Here's how the part is built. I have some questions about the finished solid (model axes, mm). Face numbers are marked on the shaded views. A direction names the side the tool comes from. Coordinates: 2 decimals unless noted, no trailing zeros. Write each loop counter-clockwise with the first axis right and the second up, starting at its lowest first coordinate (ties: lowest second). Pieces come first, ordered by that corner, then holes. Notation, with made-up numbers: M 35.25,24.25 L 58.25,24.25 A17 cw 58.25,42.25 Z; hole C 68,65 d2. An arc over 180 degrees is marked long. Use one line per item in the form item = value. Start each with the question number.
1. I'm going to push flat-ended pins straight in: pin 1 Ø5 at (x, y) = (365, -1) entering from +Z; pin 2 Ø3 at (x, z) = (369.5, 5.5) entering from -Y; pin 3 Ø3 at (x, z) = (371.5, 0.5) entering from -Y; pin 4 Ø3 at (x, y) = (354, -3.5) entering from +Z. Where does each tip first touch, or does it pass through?
2. On a 3-axis mill with a long thin cutter (end or side, diameter ignored), from which of +Z, -Z, +X, -X, +Y, -Y can I reach the whole of each face in a straight line? I mean the marked faces 5, 6 and 7. Say none if no direction works.
3. I want a section at B-B, the plane x = 351.5. List the corners of the cut face in (y, z) for me, plus the area to 3 significant figures.
4. I want a section at C-C, the plane x = 344. List the corners of the cut face in (y, z) for me, plus the area to 3 significant figures.
5. Thinking about a two-plate mould opening in Z: for the marked faces 1, 2, 3 and 4, which applies, released by +Z, released by -Z, zero draft, split by the parting line, or undercut?
6. Please list where these lines run through material, in increasing order: line 1 along X through (y, z) = (0, 0); line 2 along Y through (x, z) = (339.25, 0); line 3 along X through (y, z) = (1.75, -4.5). Write a range as [from, to].
7. I want a section at A-A, the plane z = 0. Count the separate pieces of the cut face and the enclosed holes in it, plus the area to 3 significant figures.
from build123d import *

# Parameters (mm, degrees)
SKETCH1_R               = 143.51
BOSS_EXTRUDE1_DEPTH     = 50.8
SKETCH2_R               = 68.58
BOSS_EXTRUDE2_DEPTH     = 838.2
CUT_EXTRUDE1_DEPTH      = 912.872381532
CUT_EXTRUDE1_DEPTH_BACK = 912.872381532
SKETCH3_W               = 604.52
SKETCH3_H               = 58.42
SKETCH4_R               = 50.8
CUT_EXTRUDE2_DEPTH      = 236.22
SKETCH5_W               = 63.5
SKETCH5_H               = 19.05
BOSS_EXTRUDE3_DEPTH     = 29.21
FILLET1_R               = 25.4
SCALE1_SCALE            = 0.05


with BuildPart() as part:
    # Sketch1 → Boss-Extrude1 (new body)
    with BuildSketch(Plane(origin=(0, 0, 0), x_dir=(0, 0, -1), z_dir=(1, 0, 0))):
        Circle(SKETCH1_R)
    extrude(amount=BOSS_EXTRUDE1_DEPTH)

    # Sketch2 → Boss-Extrude2 (add)
    with BuildSketch(Plane(origin=(50.8, 0, 0), x_dir=(0, 0, -1), z_dir=(1, 0, 0))):
        Circle(SKETCH2_R)
    extrude(amount=BOSS_EXTRUDE2_DEPTH)

    # Sketch3 → Cut-Extrude1 (cut, two sides: drawn at the far end of the back side and taken through both)
    with BuildSketch(Plane(origin=(0, 0, 0), x_dir=(1, 0, 0), z_dir=(0, 1, 0)).offset(-CUT_EXTRUDE1_DEPTH_BACK)):
        with Locations((556.26, 0)):
            Rectangle(SKETCH3_W, SKETCH3_H)
    extrude(amount=CUT_EXTRUDE1_DEPTH + CUT_EXTRUDE1_DEPTH_BACK, mode=Mode.SUBTRACT)

    # Sketch4 → Cut-Extrude2 (cut)
    with BuildSketch(Plane.ZY):
        Circle(SKETCH4_R)
    extrude(amount=-CUT_EXTRUDE2_DEPTH, mode=Mode.SUBTRACT)

    # Sketch5 → Boss-Extrude3 (add, symmetric)
    with BuildSketch(Plane.XY):
        with Locations((788.67, 52.523306182)):
            Rectangle(SKETCH5_W, SKETCH5_H)
    extrude(amount=BOSS_EXTRUDE3_DEPTH, both=True)

    # Fillet1
    fillet1_edges = [part.edges().sort_by_distance(p)[0] for p in [
        (0, 0, 143.51),
        (50.8, 0, 143.51),
    ]]
    fillet(fillet1_edges, radius=FILLET1_R - 0.0001)  # a hair under: the kernel refuses the full size


with BuildPart() as part_1:
    # Scale1: scaled about (350.332507714, 0.417323247, 0)
    add(part.part.scale(SCALE1_SCALE).moved(Location((332.815882328, 0.396457085, 0))))


solid = part_1.part
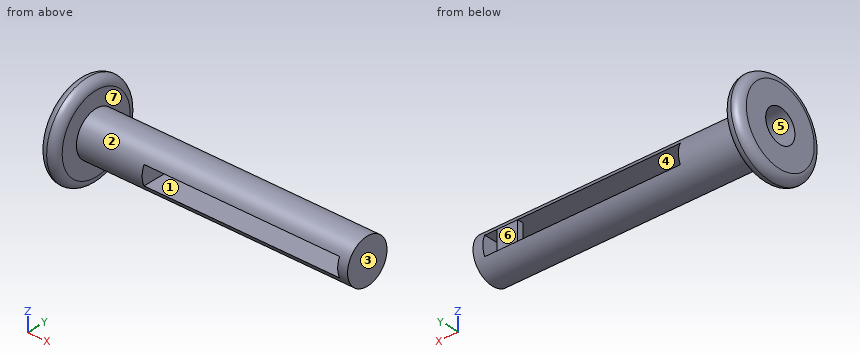
Answer list:
q1.pin_1 = 3.43
q1.pin_2 = through
q1.pin_3 = -2.71
q1.pin_4 = 2.45
q2.face_5 = -X
q2.face_6 = +Z, -Z, +Y
q2.face_7 = +X
q3.outline = M -2.71,-1.46 A3.43 ccw 3.5,-1.46 Z; M -2.71,1.46 L 3.5,1.46 A3.43 ccw Z
q3.area = 17.5 mm²
q4.outline = C 0.4,0 d6.86; hole C 0.4,0 d5.08
q4.area = 16.7 mm²
q5.face_1 = undercut
q5.face_2 = split by the parting line
q5.face_3 = zero draft
q5.face_4 = undercut
q6.line_1 = [344.63, 345.52], [375.74, 377.27]
q6.line_2 = [-3.03, -2.14], [2.94, 3.83]
q6.line_3 = [332.82, 335.36]
q7.separate_pieces = 3
q7.enclosed_holes = 0
q7.area = 58.2 mm²
